```python
from build123d import *

# Parameters (mm, degrees)
F0_R     = 15
F0_R_2   = 13.8
F1_DEPTH = 5
F2_R     = 15
F2_R_2   = 13.8
F3_DEPTH = 80
F4_R     = 15
F4_R_2   = 13.8
F4_R_3   = 11.8
F5_DEPTH = 5


with BuildPart() as f1:
    # F0 (on Right) → F1 (new body)
    with BuildSketch(Plane.YZ):
        Circle(F0_R)
        Circle(F0_R_2, mode=Mode.SUBTRACT)
        Circle(F0_R_2)
    extrude(amount=F1_DEPTH)

    # F2 (on face) → F3 (join)
    with BuildSketch(Plane.YZ.offset(5)):
        Circle(F2_R)
        Circle(F2_R_2, mode=Mode.SUBTRACT)
    extrude(amount=F3_DEPTH)

    # F4 (on face) → F5 (join)
    with BuildSketch(Plane.YZ.offset(85)):
        Circle(F4_R)
        Circle(F4_R_2, mode=Mode.SUBTRACT)
        Circle(F4_R_2)
        Circle(F4_R_3, mode=Mode.SUBTRACT)
    extrude(amount=F5_DEPTH)


solid = f1.part
```
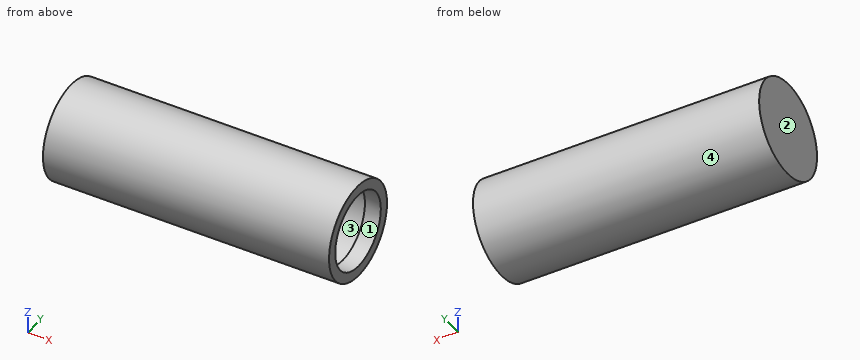
The listing builds one solid part. Answer for the finished solid, in the listing's coordinates (mm). Face numbers are marked on the shaded views. Coordinates: 2 decimals unless noted, no trailing zeros. Loops run counter-clockwise (first coordinate to the right, second up) from the corner with the lowest first, then second, coordinate; pieces in that order, holes last. Notation, with made-up numbers: (-29.5, -8) - (15.5, -8) arc R13 ccw to (15.5, -1) - close; hole circle Ø7 at (-27, 84.25). An arc over 180 degrees is marked (long way). Write item = value, one per line.
1) Determine the mould class of the marked faces 1, 2, 3 and 4 for opening direction Y: pulls with the +Y half, pulls with the -Y half, needs draft (parallel to the pull), parting line crosses it, or undercut.
Responses:
face_1 = undercut
face_2 = needs draft
face_3 = undercut
face_4 = parting line crosses it
2) Section C-C (x = 69.5) is taken. Determine the outline of the cut face in (y, z).
Responses:
outline = circle Ø30 at (0, 0); hole circle Ø27.6 at (0, 0)
3) Section A-A (y = 0) is taken. Determine the outline of the cut face in (x, z), plus the area to 3 significant figures.
Responses:
outline = (0, -15) - (90, -15) - (90, -11.8) - (85, -11.8) - (85, -13.8) - (5, -13.8) - (5, 13.8) - (85, 13.8) - (85, 11.8) - (90, 11.8) - (90, 15) - (0, 15) - close
area = 374 mm^2
4) Find the intervals of material crossed by line 1 along X through (y, z) = (-0.5, 13.75); line 2 along Z through (x, y) = (86.55, 0); line 3 along Y through (x, z) = (84.5, -5.75), in increasing order.
Responses:
line_1 = 0 to 5, 85 to 90
line_2 = -15 to -11.8, 11.8 to 15
line_3 = -13.85 to -12.55, 12.55 to 13.85
5) Each of these flat-tipped pins is pushed along its axis until it touches: P1, Ø3, axis at x = 24.5, y = -5.5, coming from the -Z side; P2, Ø4, axis at x = 9.5, y = 3, coming from the +Z side; P3, Ø5, axis at x = 34.5, z = 11, coming from the +Y side. Where does it stop, or does it pass through?
Responses:
P1 = -14.46
P2 = 14.97
P3 = 12.36
